```python
from build123d import *

# Parameters (mm, degrees)
F1_DEPTH = 6.35


with BuildPart() as f1:
    # F0 (on Front) → F1 (new body)
    with BuildSketch(Plane.XZ):
        Polygon((34.925, 18.654233), (0, 4.931788), (0, 0), (0, -2.688212), (27.305, 7.549116), (27.305, -6.668439), (0, -16.905767), (0, -24.525767), (34.925, -10.803323), align=None)
        Polygon((0, 0), (0, 4.931788), (-34.925, 18.654233), (-34.925, -10.803323), (0, -24.525767), (0, -16.905767), (-27.305, -6.668439), (-27.305, 7.549116), (0, -2.688212), align=None)
    extrude(amount=F1_DEPTH)


solid = f1.part
```
CAD build for the part. Positions are in the model's coordinates, mm. A direction names the side the tool comes from. Round coordinates to 2 decimals unless told otherwise and drop trailing zeros. Loops run counter-clockwise (first coordinate to the right, second up) from the corner with the lowest first, then second, coordinate; pieces in that order, holes last. Notation, with made-up numbers: M 84.25,-4.5 L 126.25,-4.5 A25 cw 126.25,15.5 Z; hole C 19,34.5 d9. An arc over 180 degrees is marked long. Return JSON: item names as keys, results as strings. Group by question number.
(1) Mould opens along X. For faces 4 (the flat face through (-13.46, -3.13, -11.86)), 5 (the flat face through (-27.305, -3, 0)), 6 (the flat face through (-34.925, -3, 4)), 7 (the flat face through (17.22, -3.13, -17.76)) say: +X half, -X half, draft (parallel to the pull), parting line (faces both ways), or undercut.
(2) Tool access for faces 1 (the flat face through (-17.707, -3.131, -17.568)), 2 (the flat face through (-13.84, -3.13, 2.5)), 3 (the flat face through (17.71, -3.13, 11.89)): list every direction of +Z, -Z, +X, -X, +Y, -Y with a clear straight run to the whole face (end or side of a thin tool).
(3) Saw through at B-B, the plane z = -6. List the corners of the cut face in (x, y) (3 decimals).
(4) Wall check: probe 1 along Z at (x, y) = (-24, -1); probe 2 along Z at (x, y) = (27, -3.5); probe 3 along Z at (x, y) = (31.5, -5.75). Give the ranges that are in metal, low to high. Write a range as [from, to].
(5) Saw through at A-A, the plane y = -3. List the corners of the cut face in (x, z) (3 decimals).
(6) Saw through at D-D, the plane z = -20. List the corners of the cut face in (x, y).
(7) Saw through at C-C, the plane x = 25. List the corners of the cut face in (y, z).
(8) Drop flat-ended pins along their axis: P1, Ø2, axis at x = 23, y = -5, coming from the +Z side; P2, Ø1.5, axis at x = 2, y = -4, coming from the -Z side. Give the stop position or say it passes through.
Answer list:
{
 "1": {"face 4": "undercut", "face 5": "undercut", "face 6": "-X half", "face 7": "+X half"},
 "2": {"face 1": "-Z, -X, +Y, -Y", "face 2": "+Y, -Y", "face 3": "+Z, +Y, -Y"},
 "3": {"outline": "M -34.925,-6.35 L -27.305,-6.35 L -27.305,0 L -34.925,0 Z; M 27.305,-6.35 L 34.925,-6.35 L 34.925,0 L 27.305,0 Z"},
 "4": {"probe 1": "[-15.1, -7.91], [6.31, 14.36]", "probe 2": "[-13.92, -6.78], [7.43, 15.54]", "probe 3": "[-12.15, 17.31]"},
 "5": {"outline": "M -34.925,-10.803 L 0,-24.526 L 34.925,-10.803 L 34.925,18.654 L 0,4.932 L -34.925,18.654 Z; hole M -27.305,-6.668 L 0,-16.906 L 27.305,-6.668 L 27.305,7.549 L 0,-2.688 L -27.305,7.549 Z"},
 "6": {"outline": "M -11.52,-6.35 L 11.52,-6.35 L 11.52,0 L -11.52,0 Z"},
 "7": {"outline": "M -6.35,-14.7 L 0,-14.7 L 0,-7.53 L -6.35,-7.53 Z; M -6.35,6.68 L 0,6.68 L 0,14.75 L -6.35,14.75 Z"},
 "8": {"P1": "z = 14.36", "P2": "z = -24.03"}
}
